Job drawing, mm, ordinate dimensions from the low corner. One solid piece. A direction names the side the tool comes from. Round coordinates to 2 decimals unless told otherwise and drop trailing zeros. Write each loop counter-clockwise with the first axis right and the second up, starting at its lowest first coordinate (ties: lowest second). Pieces come first, ordered by that corner, then holes.
1) Saw through at C-C (y = 29.1). Write the cut outline in (x, z), plus the area to 3 significant figures.
2) Saw through at A-A (y = 6). Write the cut outline in (x, z).
3) Saw through at D-D (z = 2). State how many separate pieces and enclosed holes the cut face has, plus the area to 3 significant figures.
4) Saw through at B-B (x = 8). Write the cut outline in (y, z).
5) Flat gauge pins, fed straight in: pin 1 (1 mm diameter, centred on x = 6.5, z = 1.5, fed in from -Y); pin 2 (2 mm diameter, centred on x = 8, y = 29.1, fed in from +Z). Where does each tip first touch, or does it go through?
6) Which spindle directions (+Z, -Z, +X, -X, +Y, -Y) get a long thin tool onto all of the face, cutting with end or side? Do the marked faces 1 and 2. Say none if no direction does.
7) Wall check: probe 1 along X at (y, z) = (6, 0.7); probe 2 along X at (y, z) = (29.1, 1.6); probe 3 along Y at (x, z) = (8, 1.9). Give the ranges that are in metal, low to high.
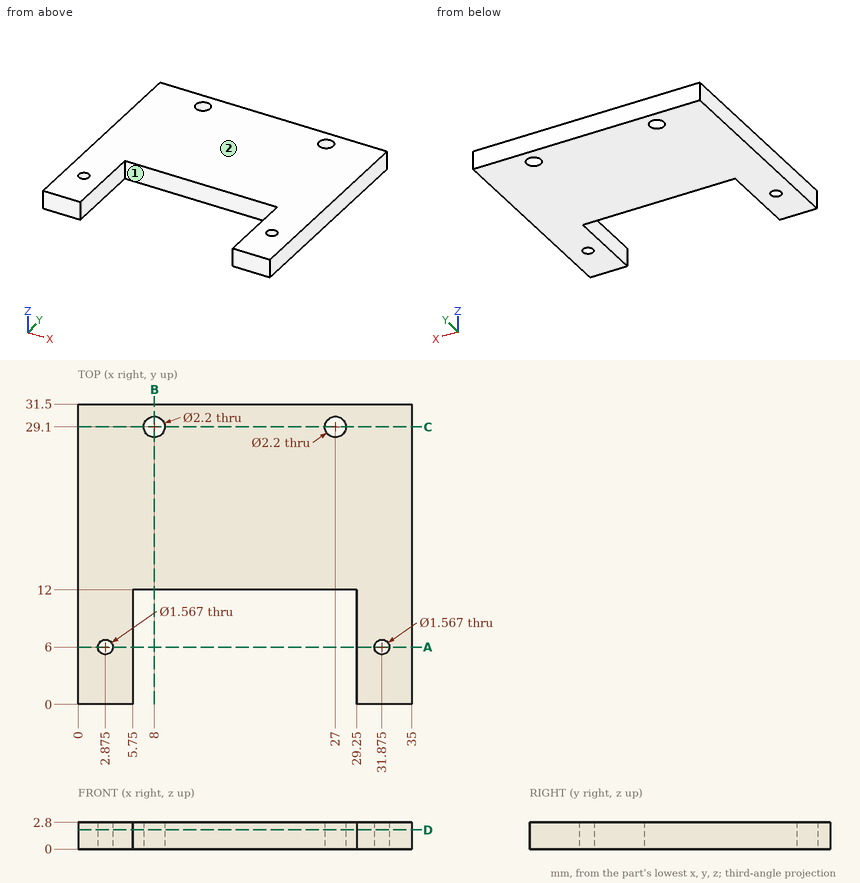
Evaluation:
1. outline: (0, 0) - (6.9, 0) - (6.9, 2.8) - (0, 2.8) - close; (9.1, 0) - (25.9, 0) - (25.9, 2.8) - (9.1, 2.8) - close; (28.1, 0) - (35, 0) - (35, 2.8) - (28.1, 2.8) - close
1. area: 85.7 mm2
2. outline: (0, 0) - (2.09, 0) - (2.09, 2.8) - (0, 2.8) - close; (3.66, 0) - (5.75, 0) - (5.75, 2.8) - (3.66, 2.8) - close; (29.25, 0) - (31.09, 0) - (31.09, 2.8) - (29.25, 2.8) - close; (32.66, 0) - (35, 0) - (35, 2.8) - (32.66, 2.8) - close
3. separate pieces: 1
3. enclosed holes: 4
3. area: 809 mm2
4. outline: (12, 0) - (28, 0) - (28, 2.8) - (12, 2.8) - close; (30.2, 0) - (31.5, 0) - (31.5, 2.8) - (30.2, 2.8) - close
5. pin 1: stops at y = 12
5. pin 2: passes through
6. face 1: +Z, -Z, -Y
6. face 2: +Z, +X, -X, +Y, -Y
7. probe 1: x = 0 to 2.09, 3.66 to 5.75, 29.25 to 31.09, 32.66 to 35
7. probe 2: x = 0 to 6.9, 9.1 to 25.9, 28.1 to 35
7. probe 3: y = 12 to 28, 30.2 to 31.5
